Geometry check sheet. Reference: the model listing, model coordinates, mm. Face numbers are marked on the shaded views. A direction names the side the tool comes from. Coordinates: 2 decimals unless noted, no trailing zeros. Order: outer loops, then holes, each group sorted by start corner. A loop starts at its lowest first (then second) coordinate and runs counter-clockwise, first axis right, second up. Notation, with made-up numbers: (4, -8) - (63, -8) arc R18 ccw to (63, 14) - close; hole circle Ø7 at (47.25, -21). An arc over 180 degrees is marked (long way). Return JSON: item names as keys, results as strings. Group by question number.
Item 1: Scan lines: probe 1 along X at (y, z) = (0, 5.55); probe 2 along X at (y, z) = (0, 6.6); probe 3 along Y at (x, z) = (1, 2). Record each from-to range of solid material in increasing order.
Item 2: Gauge pin test, flat ends, axial feed: pin 1 (1.5 mm diameter, centred on x = 0.5, y = -1.5, fed in from -Z); pin 2 (4 mm diameter, centred on x = 3, z = 6.5, fed in from -Y); pin 3 (4 mm diameter, centred on x = 1.5, z = 7, fed in from +Y); pin 4 (2 mm diameter, centred on x = 2, y = 1.5, fed in from +Z). Record the tip position at first contact, or that the pin passes through.
Item 3: Tool access check on the marked faces 4 and 5. Record the directions out of +Z, -Z, +X, -X, +Y, -Y that give a thin tool (end or side, any length) a straight path to the whole face; none if there is none.
Item 4: Draft check along Y on the marked faces 1, 2 and 3. Enter one of: pulls with the +Y half, pulls with the -Y half, needs draft (parallel to the pull), parting line crosses it, or undercut.
Item 5: Section check A-A on z = 3.25. Enter the section's corners in (x, y), then the cut area to 3 significant figures.
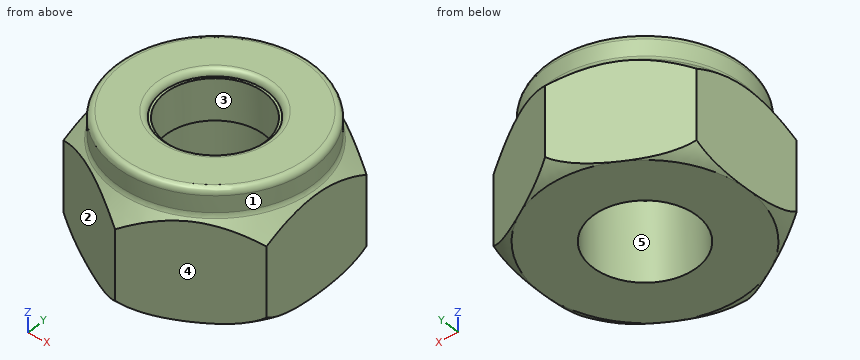
Autodesk Inventor part; units mm, degrees
ref_plane "YZ Plane" through (0, 0, 0) normal (1, 0, 0) x (0, 1, 0)
ref_plane "XZ Plane" through (0, 0, 0) normal (0, 1, 0) x (-1, 0, 0)
ref_plane "XY Plane" through (0, 0, 0) normal (0, 0, 1) x (1, 0, 0)
sketch "Sketch1" plane through (0, 0, 0) normal (0, 0, 1) x (1, 0, 0)
  line L0 (0, 7.3323) -> (6.35, 3.6662)
  line L1 (6.35, 3.6662) -> (6.35, -3.6662)
  line L2 (6.35, -3.6662) -> (0, -7.3323)
  line L3 (0, -7.3323) -> (-6.35, -3.6662)
  line L4 (-6.35, -3.6662) -> (-6.35, 3.6662)
  line L5 (-6.35, 3.6662) -> (0, 7.3323)
  line L6 (0, 10.2653) -> (0, -10.2653)
  line L7 (-8.89, 0) -> (8.89, 0)
  point P0 (0, 0)
  dimension "d0" = 12.7
extrude "Extrusion1" add sketch "Sketch1" along normal blind 7.8486
sketch "Sketch2" plane through (0, 0, 0) normal (1, 0, 0) x (0, 1, 0)
  line L0 (7.3323, 0) -> (7.3323, 7.8486)
  line L1 (3.6662, 7.8486) -> (-3.6662, 7.8486)
  line L2 (7.3323, 7.8486) -> (3.6662, 7.8486)
  line L3 (3.6662, 7.8486) -> (7.3323, 7.8486)
  line L4 (-3.6662, 7.8486) -> (3.6662, 7.8486)
  line L5 (-7.3323, 7.8486) -> (-3.6662, 7.8486)
  line L6 (-3.6662, 7.8486) -> (-7.3323, 7.8486)
  line L7 (7.3323, 5.0546) -> (6.096, 6.2909)
  line L8 (6.096, 6.2909) -> (6.096, 7.8486)
  line L9 (7.3323, 7.8486) -> (7.3323, 5.0546)
  line L10 (5.588, 7.4676) -> (3.048, 7.4676)
  line L11 (3.048, 7.4676) -> (3.048, 4.9276)
  line L12 (3.048, 4.9276) -> (5.588, 4.9276)
  line L13 (5.588, 4.9276) -> (5.588, 7.4676)
  line L14 (0, 13.9621) -> (0, -2.3404)
  arc A0 (6.35, 0) -> (7.3323, 0.762) centre (5.3317, 2.327) ccw
  line L15 (7.3323, 0) -> (3.6662, 0)
  line L16 (6.35, 0) -> (7.3323, 0)
  line L17 (7.3323, 0.762) -> (7.3323, 0)
  dimension "d3" = 2.794
  dimension "d4" = 45
  dimension "d5" = 6.096
  dimension "d6" = 3.048
  dimension "d7" = 0.381
  dimension "d8" = 2.54
  dimension "d9" = 2.54
  dimension "d11" = 6.35
  dimension "d12" = 0.762
  dimension "d13" = 2.54
revolve "Revolution1" cut sketch "Sketch2" angle 360 about axis through (0, 0, 0) along (0, 0, -1) contours L7 L8 L2 L0
revolve "Revolution2" cut sketch "Sketch2" angle 360 about axis through (0, 0, 0) along (0, 0, -1) contours L15 A0 L0
hole "Hole1" at (0, 0, 7.8486) direction (0, 0, -1) diameter 6.4008 end through all
fillet "Fillet1" radius 0.381 3 edges at (0, -6.096, 6.2909) (0, -6.096, 7.8486) (0, 3.2004, 7.8486)
revolve "Revolution3" add sketch "Sketch2" angle 360 about axis through (0, 0, 0) along (0, 0, -1) contours L13 L12 L11 L10
properties part number "HW-00033" material "Steel"
Computed:
{
 "1": {"probe 1": "x = -6.35 to -3.05, 3.05 to 6.35", "probe 2": "x = -6.1 to -3.05, 3.05 to 6.1", "probe 3": "y = -6.75 to -3.04, 3.04 to 6.75"},
 "2": {"pin 1": "passes through", "pin 2": "stops at y = -6.64", "pin 3": "stops at y = 7.07", "pin 4": "stops at z = 7.84"},
 "3": {"face 4": "+Z, -Z, +X, -Y", "face 5": "-Z"},
 "4": {"face 1": "parting line crosses it", "face 2": "pulls with the -Y half", "face 3": "undercut"},
 "5": {"outline": "(-6.35, -3.67) - (0, -7.33) - (6.35, -3.67) - (6.35, 3.67) - (0, 7.33) - (-6.35, 3.67) - close; hole circle Ø6.4 at (0, 0)", "area": "108 mm²"}
}
